from build123d import *

# Parameters (mm, degrees)
SKETCH_1_W          = 54.99998652
SKETCH_1_H          = 95.00001066
EXTRUDE_1_DEPTH     = 1
SKETCH_3_W          = 7.5000204
SKETCH_3_H          = 5
SKETCH_3_W_2        = 9.99999
SKETCH_3_W_3        = 14.99998
SKETCH_3_W_4        = 11.2500256
SKETCH_3_W_5        = 8.7500052
SKETCH_3_W_6        = 6.2500356
SKETCH_3_W_7        = 6.2499848
CUT_EXTRUDE_1_DEPTH = 1
SKETCH_7_R          = 1.75
CUT_EXTRUDE_4_DEPTH = 1
SKETCH_8_W          = 54.99998652
SKETCH_8_H          = 1
EXTRUDE_2_DEPTH     = 5
SKETCH_9_W          = 54.99998652
SKETCH_9_H          = 1
EXTRUDE_3_DEPTH     = 5
SKETCH_10_W         = 1
SKETCH_10_H         = 105.00001066
EXTRUDE_4_DEPTH     = 5
SKETCH_11_W         = 1
SKETCH_11_H         = 105.00001066
EXTRUDE_5_DEPTH     = 5


with BuildPart() as part:
    # 草图1 → 凸台-拉伸1 (new body)
    with BuildSketch(Plane.XY):
        with Locations((52.49999406, 77.49999359)):
            Rectangle(SKETCH_1_W, SKETCH_1_H)
    extrude(amount=EXTRUDE_1_DEPTH)

    # 草图3 → 切除-拉伸1 (cut)
    with BuildSketch(Plane.XY.offset(1)):
        with Locations((75.7119898, 115.57)):
            Rectangle(SKETCH_3_W, SKETCH_3_H)
        with Locations((74.462005, 108.966)):
            Rectangle(SKETCH_3_W_2, SKETCH_3_H)
        with Locations((71.96201254, 101.346)):
            Rectangle(SKETCH_3_W_3, SKETCH_3_H)
        with Locations((73.8089964, 93.726)):
            Rectangle(SKETCH_3_W_4, SKETCH_3_H)
        with Locations((72.5790014, 85.852)):
            Rectangle(SKETCH_3_W_5, SKETCH_3_H)
        with Locations((73.8089964, 78.5831296)):
            Rectangle(SKETCH_3_W_4, SKETCH_3_H)
        with Locations((72.5680286, 71.0116944)):
            Rectangle(SKETCH_3_W_5, SKETCH_3_H)
        with Locations((73.8089964, 63.44031)):
            Rectangle(SKETCH_3_W_4, SKETCH_3_H)
        with Locations((72.5680286, 55.8688748)):
            Rectangle(SKETCH_3_W_5, SKETCH_3_H)
        with Locations((73.8089964, 48.2974396)):
            Rectangle(SKETCH_3_W_4, SKETCH_3_H)
        with Locations((72.5680286, 40.7260044)):
            Rectangle(SKETCH_3_W_5, SKETCH_3_H)
        with Locations((37.440997, 84.1740252)):
            Rectangle(SKETCH_3_W_6, SKETCH_3_H)
        with Locations((28.4409896, 84.1740252)):
            Rectangle(SKETCH_3_W_7, SKETCH_3_H)
        with Locations((37.440997, 76.6740148)):
            Rectangle(SKETCH_3_W_6, SKETCH_3_H)
        with Locations((28.4409896, 76.6740148)):
            Rectangle(SKETCH_3_W_7, SKETCH_3_H)
        with Locations((37.440997, 69.1740044)):
            Rectangle(SKETCH_3_W_6, SKETCH_3_H)
        with Locations((28.4409896, 69.1740044)):
            Rectangle(SKETCH_3_W_7, SKETCH_3_H)
        with Locations((37.440997, 61.673994)):
            Rectangle(SKETCH_3_W_6, SKETCH_3_H)
        with Locations((28.4409896, 61.673994)):
            Rectangle(SKETCH_3_W_7, SKETCH_3_H)
        with Locations((37.440997, 54.1739836)):
            Rectangle(SKETCH_3_W_6, SKETCH_3_H)
        with Locations((28.4409896, 54.1739836)):
            Rectangle(SKETCH_3_W_7, SKETCH_3_H)
        with Locations((37.440997, 46.674024)):
            Rectangle(SKETCH_3_W_6, SKETCH_3_H)
        with Locations((28.4409896, 46.674024)):
            Rectangle(SKETCH_3_W_7, SKETCH_3_H)
        with Locations((37.440997, 39.1740136)):
            Rectangle(SKETCH_3_W_6, SKETCH_3_H)
        with Locations((28.4409896, 39.1740136)):
            Rectangle(SKETCH_3_W_7, SKETCH_3_H)
    extrude(amount=-CUT_EXTRUDE_1_DEPTH, mode=Mode.SUBTRACT)

    # 草图7 → 切除-拉伸4 (cut)
    with BuildSketch(Plane.XY.offset(1)):
        with Locations((77.00000094, 121.99999984)):
            Circle(SKETCH_7_R)
        with Locations((27.99999988, 121.99999984)):
            Circle(SKETCH_7_R)
        with Locations((77.00000094, 33.00000004)):
            Circle(SKETCH_7_R)
        with Locations((27.9999948, 32.9999848)):
            Circle(SKETCH_7_R)
    extrude(amount=-CUT_EXTRUDE_4_DEPTH, mode=Mode.SUBTRACT)

    # 草图8 → 凸台-拉伸2 (add)
    with BuildSketch(Plane(origin=(0, 124.99999892, 0), x_dir=(1, 0, 0), z_dir=(0, 1, 0))):
        with Locations((52.49999406, -0.5)):
            Rectangle(SKETCH_8_W, SKETCH_8_H)
    extrude(amount=EXTRUDE_2_DEPTH)

    # 草图9 → 凸台-拉伸3 (add)
    with BuildSketch(Plane.XZ.offset(-29.99998826)):
        with Locations((52.49999406, 0.5)):
            Rectangle(SKETCH_9_W, SKETCH_9_H)
    extrude(amount=EXTRUDE_3_DEPTH)

    # 草图10 → 凸台-拉伸4 (add)
    with BuildSketch(Plane.ZY.offset(-25.0000008)):
        with Locations((0.5, 77.49999359)):
            Rectangle(SKETCH_10_W, SKETCH_10_H)
    extrude(amount=EXTRUDE_4_DEPTH)

    # 草图11 → 凸台-拉伸5 (add)
    with BuildSketch(Plane(origin=(79.99998732, 0, 0), x_dir=(0, 0, -1), z_dir=(1, 0, 0))):
        with Locations((-0.5, 77.49999359)):
            Rectangle(SKETCH_11_W, SKETCH_11_H)
    extrude(amount=EXTRUDE_5_DEPTH)


solid = part.part
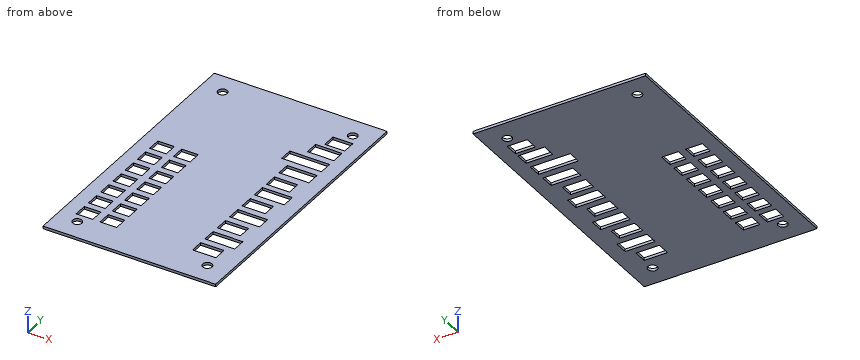
Work out the finished part from the listing and answer in its coordinate system (mm). Coordinates: 2 decimals unless noted, no trailing zeros. Loops run counter-clockwise (first coordinate to the right, second up) from the corner with the lowest first, then second, coordinate; pieces in that order, holes last. Notation, with made-up numbers: (40.5, 83) -> (49.5, 83) arc R29 cw to (49.5, 119) -> close; hole circle Ø1 at (4, 48). An arc over 180 degrees is marked (long way). Write each question's results on one line, items separated by ' | '. Start each with the question number.
1) Find section B-B on y = 70. Determine the outline of the cut face in (x, z), then the cut area to 4 significant figures.
2) Find section D-D on x = 28. Count the separate pieces of the cut face and the enclosed holes in it, then the cut area to 3 significant figures.
3) Find section A-A on x = 65.5. Determine the outline of the cut face in (y, z).
4) Consider line 1 along X through (y, z) = (55, 0.45); line 2 along X through (y, z) = (72, 0.05); line 3 along X through (y, z) = (85.5, 0.4). Determine where each line is inside the solid, lowest interval first.
5) Find section C-C on y = 116.5. Determine the outline of the cut face in (x, z).
Response values:
1) outline: (20, 0) -> (25.32, 0) -> (25.32, 1) -> (20, 1) -> close; (31.57, 0) -> (34.32, 0) -> (34.32, 1) -> (31.57, 1) -> close; (40.57, 0) -> (68.19, 0) -> (68.19, 1) -> (40.57, 1) -> close; (76.94, 0) -> (85, 0) -> (85, 1) -> (76.94, 1) -> close | area: 43.75 mm^2
2) separate pieces: 10 | enclosed holes: 0 | area: 63.0 mm^2
3) outline: (25, 0) -> (98.85, 0) -> (98.85, 1) -> (25, 1) -> close; (103.85, 0) -> (130, 0) -> (130, 1) -> (103.85, 1) -> close
4) line 1: x = 20 to 25.32, 31.57 to 34.32, 40.57 to 68.19, 76.94 to 85 | line 2: x = 20 to 68.19, 76.94 to 85 | line 3: x = 20 to 25.32, 31.57 to 34.32, 40.57 to 68.2, 76.95 to 85
5) outline: (20, 0) -> (71.96, 0) -> (71.96, 1) -> (20, 1) -> close; (79.46, 0) -> (85, 0) -> (85, 1) -> (79.46, 1) -> close
